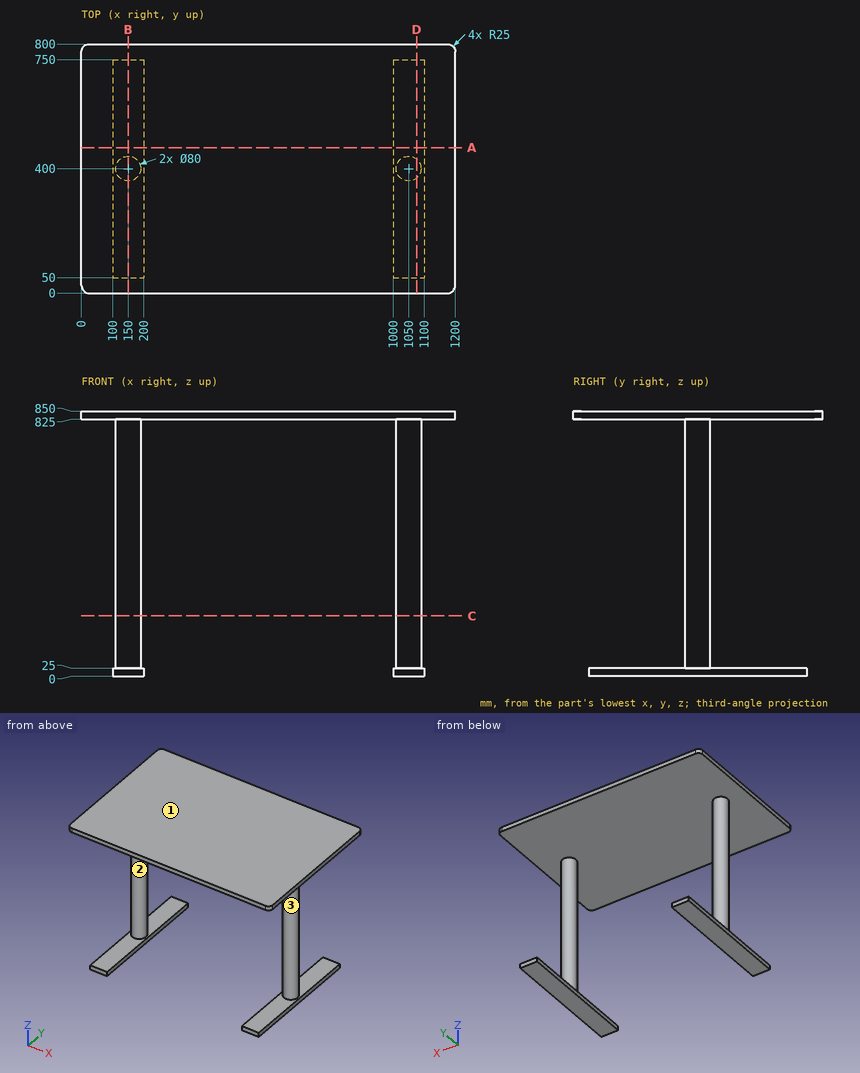
Answer from the drawing. Dimensions are ordinates in mm from the lowest x, y and z of the part. Round coordinates to 2 decimals unless told otherwise and drop trailing zeros. Write each loop counter-clockwise with the first axis right and the second up, starting at its lowest first coordinate (ties: lowest second). Pieces come first, ordered by that corner, then holes. Notation, with made-up numbers: M -20.75,29.5 L 29.25,29.5 A28 ccw 29.25,57.5 Z; hole C 4.5,-8 d8. An arc over 180 degrees is marked long. Write each question's results on one line, items separated by ' | '. Start each with the question number.
Item 1: Straight lines are drawn through the part: L1, parallel to Z at x = 159.5, y = 220.5; L2, parallel to X at y = 402, z = 72; L3, parallel to Z at x = 965, y = 676. For each, find the intervals that lie inside material, in ascending order. Write a range as [from, to].
Item 2: A cutting plane is placed at B-B on x = 150. Write down the section's boundary in (y, z), and give its area (4 significant figures).
Item 3: Flat-ended cylindrical pins translate along their axes: pin 1 Ø7.5 at (x, z) = (140, 18) entering from +Y; pin 2 Ø4 at (x, y) = (924.5, 261) entering from -Z; pin 3 Ø7.5 at (x, z) = (1047.5, 14) entering from -Y; pin 4 Ø2 at (y, z) = (441.5, 672) entering from +X. Find the tip coordinate at first contact, or state that the pin passes through.
Item 4: A cutting plane is placed at A-A on y = 467.5. Write down the section's boundary in (x, z).
Item 5: A cutting plane is placed at C-C on z = 193. Write down the section's boundary in (x, y).
Item 6: A cutting plane is placed at D-D on x = 1075.5. Write down the section's boundary in (y, z).
Item 7: For a pull along X with two mould halves and no side action, classify the marked faces 1, 2 and 3 as pulls with the +X half, pulls with the -X half, needs draft (parallel to the pull), parting line crosses it, or undercut.
Check sheet entries:
1) L1: [0, 25], [825, 850] | L2: [110.05, 189.95], [1010.05, 1089.95] | L3: [825, 850]
2) outline: M 0,825 L 360,825 L 360,25 L 50,25 L 50,0 L 750,0 L 750,25 L 440,25 L 440,825 L 800,825 L 800,850 L 0,850 Z | area: 101,500 mm²
3) pin 1: y = 750 | pin 2: z = 825 | pin 3: y = 50 | pin 4: through
4) outline: M 0,825 L 1200,825 L 1200,850 L 0,850 Z; M 100,0 L 200,0 L 200,25 L 100,25 Z; M 1000,0 L 1100,0 L 1100,25 L 1000,25 Z
5) outline: C 150,400 d80; C 1050,400 d80
6) outline: M 0,825 L 369.18,825 L 369.18,25 L 50,25 L 50,0 L 750,0 L 750,25 L 430.82,25 L 430.82,825 L 800,825 L 800,850 L 0,850 Z
7) face 1: needs draft | face 2: undercut | face 3: undercut
